Can you work these out from the model? Positions are in its coordinate system, mm. A direction names the side the tool comes from. Give positions to 0.01 mm unless a question says otherwise; leave off trailing zeros. Write each loop counter-clockwise with the first axis right and the second up, starting at its lowest first coordinate (ties: lowest second). Pieces come first, ordered by that corner, then holes.
from build123d import *

# Parameters (mm, degrees)
F0_W     = 50.8
F0_H     = 38.1
F1_DEPTH = 31.75
F2_W     = 25.4
F2_H     = 19.05
F3_DEPTH = 31.75
F5_DEPTH = 50.8


with BuildPart() as f1:
    # F0 (on Front) → F1 (new body)
    with BuildSketch(Plane.XZ):
        with Locations((25.4, 19.05)):
            Rectangle(F0_W, F0_H)
    extrude(amount=F1_DEPTH)

    # F2 (on face) → F3 (cut)
    with BuildSketch(Plane.XZ.offset(31.75)):
        with Locations((25.4, 28.575)):
            Rectangle(F2_W, F2_H)
    extrude(amount=-F3_DEPTH, mode=Mode.SUBTRACT)

    # F4 (on face) → F5 (cut)
    with BuildSketch(Plane.YZ.offset(50.8)):
        with BuildLine():
            Line((-31.75, 38.1), (-31.75, 12.7))
            ThreePointArc((-31.75, 12.7), (-14.767814, 21.117814), (-6.35, 38.1))
            Line((-6.35, 38.1), (-31.75, 38.1))
        make_face()
    extrude(amount=-F5_DEPTH, mode=Mode.SUBTRACT)


solid = f1.part
(1) Imagine slicing it at C-C, the plane y = -2.5. Write out the boundary of the cut face in (x, z), plus the area to 3 significant figures.
Returned:
outline: (0, 0) - (50.8, 0) - (50.8, 38.1) - (38.1, 38.1) - (38.1, 19.05) - (12.7, 19.05) - (12.7, 38.1) - (0, 38.1) - close
area: 1,450 mm2
(2) Imagine slicing it at A-A, the plane x = 46. Write out the boundary of the cut face in (y, z).
Returned:
outline: (-31.75, 0) - (0, 0) - (0, 38.1) - (-6.35, 38.1) arc R29.66 cw to (-31.75, 12.7) - close
(3) Will these pins go through, and if not, where does the flat tip stop? P1, Ø19, axis at x = 24.5, y = -10, coming from the +Z side; P2, Ø4, axis at x = 6, y = -11.5, coming from the +Z side.
Returned:
P1: stops at z = 19.05
P2: stops at z = 28.26
(4) Imagine slicing it at D-D, the plane z = 26.5. Write out the boundary of the cut face in (x, y).
Returned:
outline: (0, -10.51) - (12.7, -10.51) - (12.7, 0) - (0, 0) - close; (38.1, -10.51) - (50.8, -10.51) - (50.8, 0) - (38.1, 0) - close
(5) If I drill on L1, parallel to X at y = -5.5, z = 34.5; L2, parallel to Z at x = 36.5, y = -8; L3, parallel to Y at x = 40.5, z = 17.5, over which ranges is the centre line in solid material (lowest first)?
Returned:
L1: x = 0 to 12.7, 38.1 to 50.8
L2: z = 0 to 19.05
L3: y = -19.16 to 0
(6) If we mould it in two halves opening along X, with no side actions, what happens to faces 3 (the face through (38.1, -5, 26)), 4 (the face through (0, -12, 15)), 5 (the face through (44, -3, 38.1)), 6 (the face through (50.8, -12, 15))? For each: +X half, -X half, draft (parallel to the pull), parting line (faces both ways), or undercut.
Returned:
face 3: undercut
face 4: -X half
face 5: draft
face 6: +X half
(7) Imagine slicing it at B-B, the plane z = 31. Write out the boundary of the cut face in (x, y).
Returned:
outline: (0, -8.23) - (12.7, -8.23) - (12.7, 0) - (0, 0) - close; (38.1, -8.23) - (50.8, -8.23) - (50.8, 0) - (38.1, 0) - close
(8) For faces 1 (the face through (25, 0, 15)), 2 (the face through (12.7, -5, 26)), which set-ups out of +Z, -Z, +X, -X, +Y, -Y let a thin tool reach every point of the face, with its end or its side?
Returned:
face 1: +Z, -Z, +X, -X, +Y
face 2: +Z, +Y, -Y
